Part model, mm, in its own coordinate system. A direction names the side the tool comes from. Coordinates: 2 decimals unless noted, no trailing zeros. Order: outer loops, then holes, each group sorted by start corner. A loop starts at its lowest first (then second) coordinate and runs counter-clockwise, first axis right, second up. Notation, with made-up numbers: M 15.5,12.25 L 72.5,12.25 A23 ccw 72.5,21.25 Z; hole C -14,28.25 d8. An arc over 180 degrees is marked long. Write item = value, one per line. Start each with the question number.
from build123d import *

# Parameters (mm, degrees)
F1_DEPTH = 17.5
F3_D     = 4.2
F3_DEPTH = 20
F3_TIP   = 1.2618073
F5_D     = 4.2
F5_DEPTH = 17
F5_TIP   = 1.2618073


with BuildPart() as f1:
    # F0 (on Front) → F1 (new body, symmetric)
    with BuildSketch(Plane.XZ):
        with BuildLine():
            Line((24, -20), (24, 20))
            Line((24, 20), (-24, 20))
            Line((-24, 20), (-24, -20))
            Line((-24, -20), (-8.5, -20))
            Line((-8.5, -20), (-8.5, -11.187157816))
            ThreePointArc((-8.5, -11.187157816), (0, 14.05), (8.5, -11.187157816))
            Line((8.5, -11.187157816), (8.5, -20))
            Line((8.5, -20), (24, -20))
        make_face()
    extrude(amount=F1_DEPTH, both=True)

    # F3
    with Locations(Plane.XZ.offset(17.5)):
        with Locations((-13.4350288425, 13.4350288425), (-19, 0), (-13.4350288425, -13.4350288425), (13.4350288425, -13.4350288425), (19, 0), (13.4350288425, 13.4350288425)):
            Hole(F3_D / 2, depth=F3_DEPTH)
            with Locations((0, 0, -(F3_DEPTH + F3_TIP / 2))):  # 118° drill point
                Cone(0, F3_D / 2, F3_TIP, mode=Mode.SUBTRACT)

    # F5
    with Locations(Plane.XY.offset(20)):
        with Locations((-19, 11), (-19, -11), (19, -11), (19, 11)):
            Hole(F5_D / 2, depth=F5_DEPTH)
            with Locations((0, 0, -(F5_DEPTH + F5_TIP / 2))):  # 118° drill point
                Cone(0, F5_D / 2, F5_TIP, mode=Mode.SUBTRACT)


solid = f1.part
Item 1: Cut at A-A, the plane z = 8. Write the cut outline in (x, y), and give its area (3 significant figures).
Item 2: Flat gauge pins, fed straight in: pin 1 (3.5 mm diameter, centred on x = 19, z = 0, fed in from -Y); pin 2 (3.5 mm diameter, centred on x = 19, y = 11, fed in from +Z); pin 3 (6.5 mm diameter, centred on x = -19, z = 0, fed in from -Y). Where does each tip first touch, or does it go through?
Item 3: Wall check: line 1 along Y through (x, z) = (19, 6.5); line 2 along Z through (x, y) = (-15, -13.5); line 3 along X through (y, z) = (-11, 15). Give the ranges that are in metal, low to high. Write a range as [from, to].
Item 4: Cut at B-B, the plane y = 7. Write the cut outline in (x, z), and give its area (3 significant figures).
Item 5: Cut at C-C, the plane z = 16.5. Write the cut outline in (x, y), and give its area (3 significant figures).
Item 6: Pull direction X, two halves, no side cores. Call faces 1 (the conical face through (-19.364, 3.543, 0.016)), 2 (the flat face through (-24, 0, 0)), 3 (the flat face through (-6, 17.5, 14)): pulls with the +X half, pulls with the -X half, needs draft (parallel to the pull), parting line crosses it, or undercut.
Item 7: 3-axis set-ups, long thin cutter, end or side, ignore diameter. For faces 4 (the flat face through (16, 0, -20)), 5 (the flat face through (8.5, 0, -16)), 6 (the cylindrical face through (16.997, -10.369, 11.381)), 7 (the flat face through (0, 0, 20)), 8 (the cylindrical face through (16.997, -7.36, 0.631)): which of +Z, -Z, +X, -X, +Y, -Y reach the whole face in a straight line?
Item 8: Cut at D-D, the plane x = 9.5. Write the cut outline in (y, z), and give its area (3 significant figures).
Filled sheet:
q1.outline = M -24,-17.5 L -11.55,-17.5 L -11.55,17.5 L -24,17.5 Z; M 11.55,-17.5 L 24,-17.5 L 24,17.5 L 11.55,17.5 Z; hole C -19,-11 d4.2; hole C -19,11 d4.2; hole C 19,-11 d4.2; hole C 19,11 d4.2
q1.area = 816 mm2
q2.pin_1 = 2.71
q2.pin_2 = 2.79
q2.pin_3 = -17.5
q3.line_1 = [-17.5, -13.1], [-8.9, 8.9], [13.1, 17.5]
q3.line_2 = [-20, -14.84], [-12.03, 12.03], [14.84, 20]
q3.line_3 = [-24, -21.1], [-16.9, -14.84], [-12.03, 12.03], [14.84, 16.9], [21.1, 24]
q4.outline = M -24,-20 L -8.5,-20 L -8.5,-11.19 A14.05 cw long 8.5,-11.19 L 8.5,-20 L 24,-20 L 24,20 L -24,20 Z
q4.area = 1,180 mm2
q5.outline = M -24,-17.5 L 24,-17.5 L 24,17.5 L -24,17.5 Z; hole C -19,-11 d4.2; hole C -19,11 d4.2; hole C 19,-11 d4.2; hole C 19,11 d4.2
q5.area = 1,620 mm2
q6.face_1 = undercut
q6.face_2 = pulls with the -X half
q6.face_3 = needs draft
q7.face_4 = -Z, +X, -X, +Y, -Y
q7.face_5 = -Z, +Y, -Y
q7.face_6 = +Z
q7.face_7 = +Z, +X, -X, +Y, -Y
q7.face_8 = -Y
q8.outline = M -17.5,-20 L 17.5,-20 L 17.5,-10.35 L -17.5,-10.35 Z; M -17.5,10.35 L 17.5,10.35 L 17.5,20 L -17.5,20 Z
q8.area = 675 mm2
